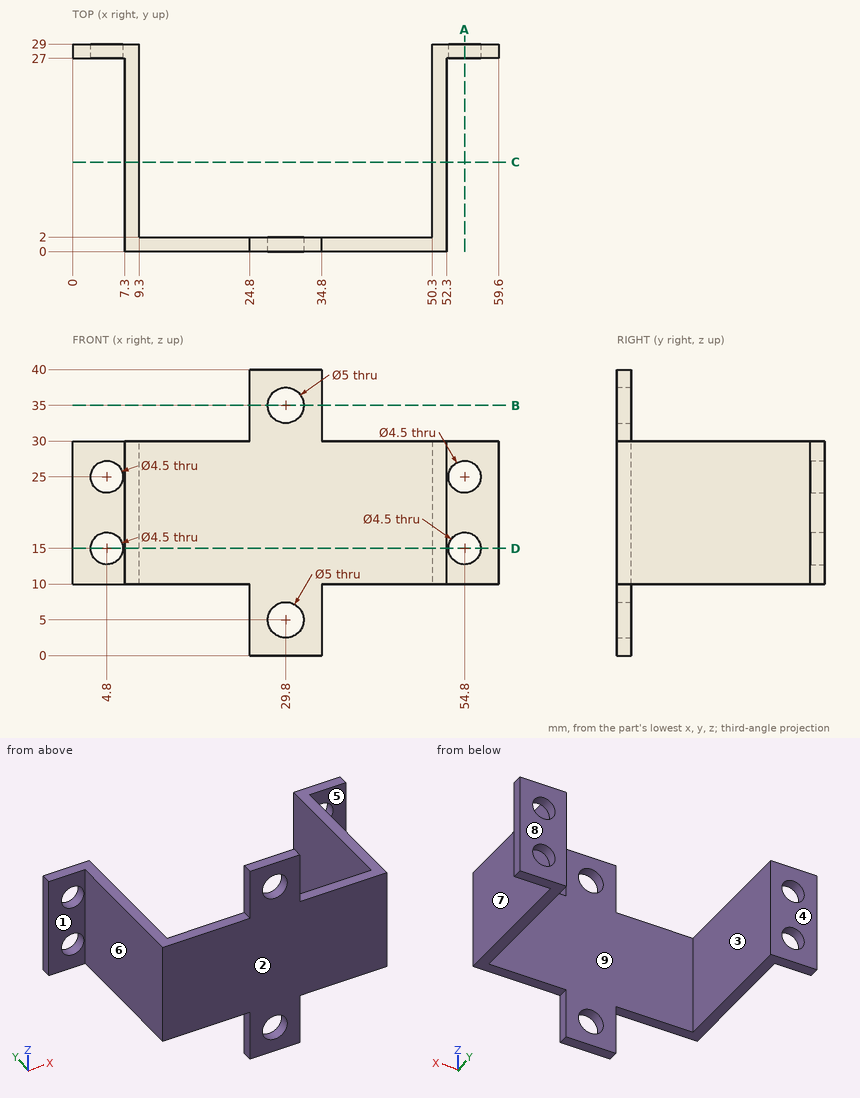
Design review of the part shown in the three views and the two pictorial views. Dimensions are in mm from the part's minimum x, y and z. A direction names the side the tool comes from. Round coordinates to 2 decimals unless told otherwise and drop trailing zeros. Write each loop counter-clockwise with the first axis right and the second up, starting at its lowest first coordinate (ties: lowest second). Pieces come first, ordered by that corner, then holes. Notation, with made-up numbers: M 57,85 L 78,85 A17 cw 78,98 Z; hole C -24,-10 d2. An arc over 180 degrees is marked long. One line per item, written item: value. Start each with the question number.
1. Take a section at A-A on x = 54.8. State the section outline as (y, z) points.
2. Draft analysis for pull direction X (two halves, no side actions). For the marked faces 6, 7, 8 and 9, state which applies: pulls with the +X half, pulls with the -X half, needs draft (parallel to the pull), parting line crosses it, or undercut.
3. Take a section at D-D on z = 15. State the section outline as (x, y) points.
4. Take a section at C-C on y = 12.5. State the section outline as (x, z) points.
5. For the marked faces 1, 2, 3, 4 and 5, list the 3-axis set-ups (+Z, -Z, +X, -X, +Y, -Y) from which the entire face can be reached by the end or side of a thin tool; tool diameter is ignored.
6. Clearance check with flat-ended pins moving along their axes: P1, Ø4, axis at y = 16, z = 22.5, coming from the +X side; P2, Ø16, axis at y = 21, z = 19, coming from the -X side; P3, Ø8, axis at x = 10.5, y = 17, coming from the +Z side; P4, Ø10, axis at y = 18.5, z = 23.5, coming from the -X side. State where each tip first meets the part, or that it passes through.
7. Take a section at B-B on z = 35. State the section outline as (x, y) points.
8. To check wall thickness, follow probe 1 along X at (y, z) = (27.5, 15); probe 2 along Z at (x, y) = (4.8, 28.55); probe 3 along Z at (x, y) = (29.8, 0.9). State the ranges of each line that lie inside material, in increasing order. Write a range as from..to.
Computed:
1. outline: M 27,10 L 29,10 L 29,12.75 L 27,12.75 Z; M 27,17.25 L 29,17.25 L 29,22.75 L 27,22.75 Z; M 27,27.25 L 29,27.25 L 29,30 L 27,30 Z
2. face 6: pulls with the -X half
2. face 7: pulls with the +X half
2. face 8: needs draft
2. face 9: undercut
3. outline: M 0,27 L 2.55,27 L 2.55,29 L 0,29 Z; M 7.05,27 L 7.3,27 L 7.3,0 L 52.3,0 L 52.3,27 L 52.55,27 L 52.55,29 L 50.3,29 L 50.3,2 L 9.3,2 L 9.3,29 L 7.05,29 Z; M 57.05,27 L 59.6,27 L 59.6,29 L 57.05,29 Z
4. outline: M 7.3,10 L 9.3,10 L 9.3,30 L 7.3,30 Z; M 50.3,10 L 52.3,10 L 52.3,30 L 50.3,30 Z
5. face 1: +Z, -Z, -X, -Y
5. face 2: +Z, -Z, +X, -X, -Y
5. face 3: +Z, -Z, +Y
5. face 4: +Z, -Z, +X, -X, +Y
5. face 5: +Z, -Z, +X, -Y
6. P1: stops at x = 52.3
6. P2: stops at x = 0
6. P3: stops at z = 30
6. P4: stops at x = 7.3
7. outline: M 24.8,0 L 27.3,0 L 27.3,2 L 24.8,2 Z; M 32.3,0 L 34.8,0 L 34.8,2 L 32.3,2 Z
8. probe 1: x = 0..2.55, 7.05..9.3, 50.3..52.55, 57.05..59.6
8. probe 2: z = 10..12.75, 17.25..22.75, 27.25..30
8. probe 3: z = 0..2.5, 7.5..32.5, 37.5..40
